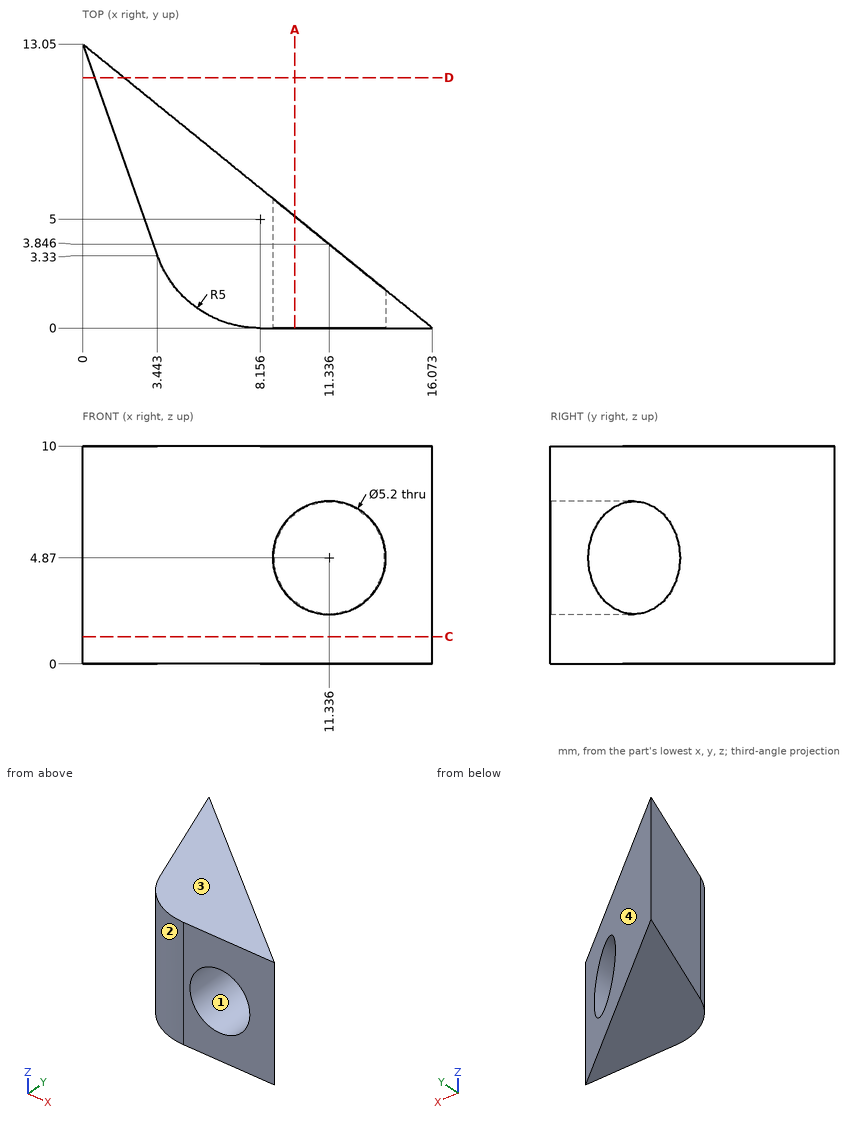
Input: dimensioned drawing with shaded views. Units: mm. Origin: part minimum x, y, z. Coordinates: 2 decimals unless noted, no trailing zeros. Order: outer loops, then holes, each group sorted by start corner. A loop starts at its lowest first (then second) coordinate and runs counter-clockwise, first axis right, second up. Notation, with made-up numbers: (82, 85.5) - (93, 85.5) arc R31 ccw to (93, 110.5) - close; hole circle Ø11 at (81, 46.5). An arc over 180 degrees is marked (long way). Return JSON: item names as keys, results as strings. Group by question number.
1. Material intervals for line 1 along X through (y, z) = (8.5, 4.25) (1 decimal); line 2 along Z through (x, y) = (11, 4); line 3 along Y through (x, z) = (12.5, 9.25), sorted ascending. Write a range as [from, to].
2. Cut plane C-C (z = 1.25). Output: boundary loops of the cut face in (x, y).
3. Pull-direction query (X, two-part tool) for the marked faces 1, 2, 3 and 4; classes: pulls with the +X half, pulls with the -X half, needs draft (parallel to the pull), parting line crosses it, or undercut.
4. Pin query (flat end, axial travel): pin 1 (1.5 mm diameter, centred on x = 5.5, z = 8, fed in from -Y); pin 2 (3 mm diameter, centred on x = 3.5, z = 3.5, fed in from -Y); pin 3 (5 mm diameter, centred on y = 4.5, z = 4, fed in from -X). Return the tip coordinate at first contact, or that it passes through.
5. Cut plane A-A (x = 9.75). Output: boundary loops of the cut face in (y, z), plus the area to 3 significant figures.
6. Cut plane D-D (y = 11.5). Output: boundary loops of the cut face in (x, z), plus the area to 3 significant figures.
Resolved:
{
 "1": {"line 1": "x = [1.6, 5.6]", "line 2": "z = [0, 2.29], [7.45, 10]", "line 3": "y = [0, 2.9]"},
 "2": {"outline": "(0, 13.05) - (3.44, 3.33) arc R5 ccw to (8.16, 0) - (16.07, 0) - close"},
 "3": {"face 1": "undercut", "face 2": "pulls with the -X half", "face 3": "needs draft", "face 4": "pulls with the +X half"},
 "4": {"pin 1": "stops at y = 0.38", "pin 2": "stops at y = 1.12", "pin 3": "stops at x = 2.14"},
 "5": {"outline": "(0, 0) - (5.13, 0) - (5.13, 2.81) - (0, 2.81) - close; (0, 6.93) - (5.13, 6.93) - (5.13, 10) - (0, 10) - close", "area": "30.2 mm²"},
 "6": {"outline": "(0.55, 0) - (1.91, 0) - (1.91, 10) - (0.55, 10) - close", "area": "13.6 mm²"}
}
